Check sheet for the drawn part. Datum: minimum x, y, z corner. Units: mm. Give positions to 0.01 mm unless a question says otherwise; leave off trailing zeros. Order: outer loops, then holes, each group sorted by start corner. A loop starts at its lowest first (then second) coordinate and runs counter-clockwise, first axis right, second up.
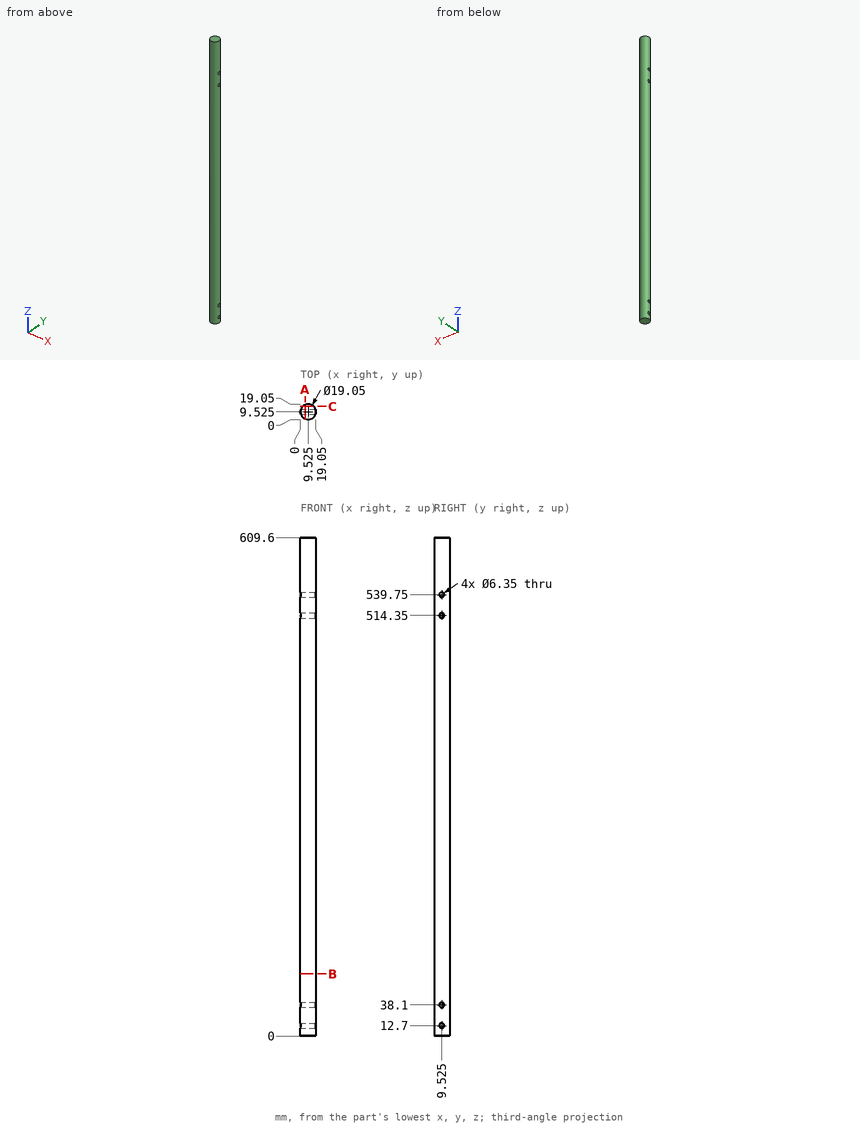
Item 1: Sectioned sample at C-C (y = 16). Enter the section's corners in (x, z).
Reported:
outline: (2.54, 0) - (16.51, 0) - (16.51, 609.6) - (2.54, 609.6) - close
Item 2: Gauge pin test, flat ends, axial feed: pin 1 (8.5 mm diameter, centred on y = 9.525, z = 38.1, fed in from +X); pin 2 (3 mm diameter, centred on y = 12.5, z = 304, fed in from -X); pin 3 (1 mm diameter, centred on x = 2, z = 142.5, fed in from +Y); pin 4 (4 mm diameter, centred on y = 9.525, z = 12.7, fed in from -X). Record the tip position at first contact, or that the pin passes through.
Reported:
pin 1: stops at x = 19.05
pin 2: stops at x = 0.11
pin 3: stops at y = 15.96
pin 4: passes through
Item 3: Sectioned sample at B-B (z = 76). Enter the section's corners in (x, y) (3 decimals).
Reported:
outline: circle Ø19.05 at (9.525, 9.525)
Item 4: Scan lines: L1, parallel to Z at x = 6.5, y = 10.25; L2, parallel to Z at x = 11.5, y = 10; L3, parallel to Y at x = 8.75, z = 12.7. Record each from-to range of solid material in increasing order.
Reported:
L1: z = 0 to 9.61, 15.79 to 35.01, 41.19 to 511.26, 517.44 to 536.66, 542.84 to 609.6
L2: z = 0 to 9.56, 15.84 to 34.96, 41.24 to 511.21, 517.49 to 536.61, 542.89 to 609.6
L3: y = 0.03 to 6.35, 12.7 to 19.02
Item 5: Sectioned sample at A-A (x = 5.75). Enter the section's corners in (y, z) (3 decimals).
Reported:
outline: (0.78, 0) - (18.27, 0) - (18.27, 609.6) - (0.78, 609.6) - close; hole circle Ø6.35 at (9.525, 12.7); hole circle Ø6.35 at (9.525, 38.1); hole circle Ø6.35 at (9.525, 514.35); hole circle Ø6.35 at (9.525, 539.75)
